The drawing under review shows one solid part. Ordinate dimensions are in mm from its lowest x, y, z. Coordinates: 2 decimals unless noted, no trailing zeros. Write each loop counter-clockwise with the first axis right and the second up, starting at its lowest first coordinate (ties: lowest second). Pieces come first, ordered by that corner, then holes. Notation, with made-up numbers: (4, 59.25) - (38, 59.25) arc R27 cw to (38, 90.25) - close; hole circle Ø11 at (49, 45). An arc over 180 degrees is marked (long way). Use a Markdown table: item, result.
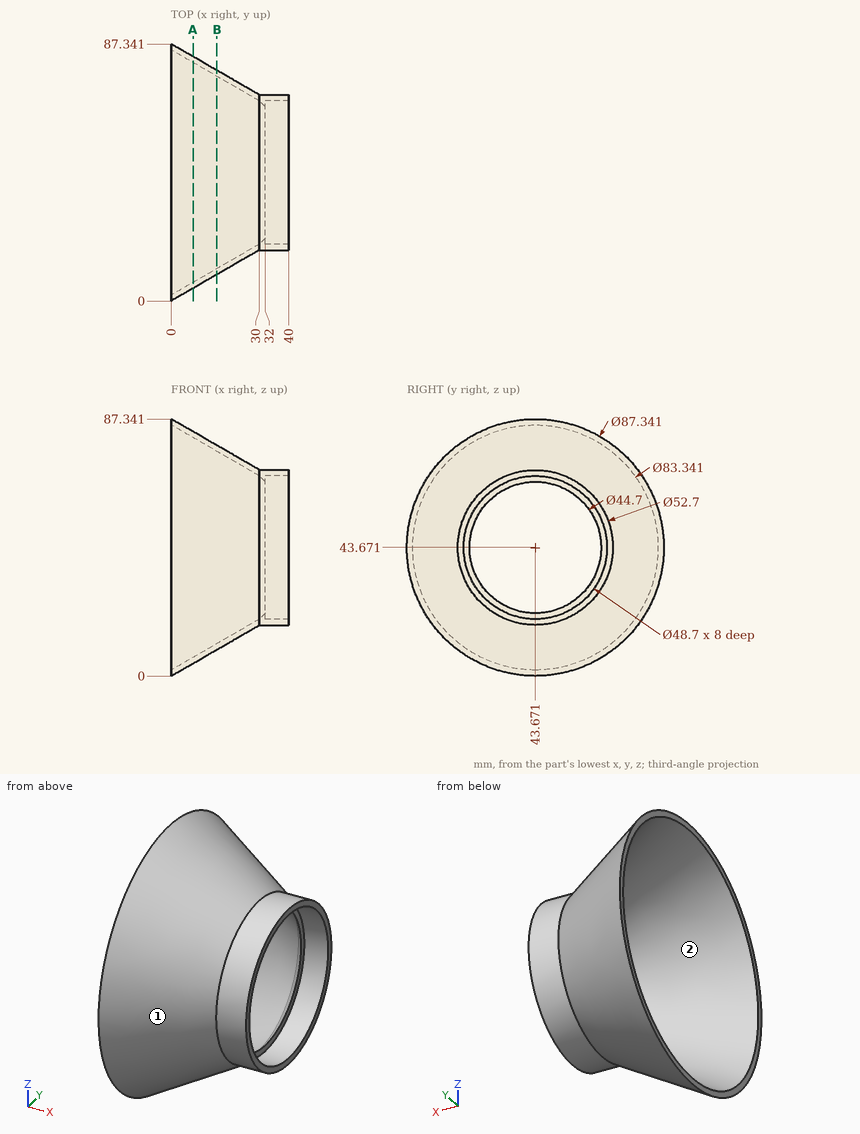
(1) For L1, parallel to Y at x = 12.5, z = 20.5 (1 decimal); L2, parallel to Y at x = 18.5, z = 47; L3, parallel to Z at x = 33, y = 58 (1 decimal), list the stretches that pass through material, from the lowest coordinate up. Write a range as from..to.
Determined:
| item | result |
|---|---|
| L1 | 15.5..18.2, 69.2..71.8 |
| L2 | 10.85..12.86, 74.48..76.49 |
| L3 | 21.6..24, 63.4..65.8 |
(2) Take a section at B-B on x = 15.5. Write out the cut boundary in (y, z).
Determined:
| item | result |
|---|---|
| outline | circle Ø69.44 at (43.67, 43.67); hole circle Ø65.44 at (43.67, 43.67) |
(3) Draft analysis for pull direction Y (two halves, no side actions). For the marked faces 1 and 2, state which applies: +Y half, -Y half, draft (parallel to the pull), parting line (faces both ways), or undercut.
Determined:
| item | result |
|---|---|
| face 1 | parting line |
| face 2 | undercut |
(4) For pin 1 (1.5 mm diameter, centred on x = 10, z = 15.5, fed in from +Y); pin 2 (1 mm diameter, centred on x = 16, y = 22.5, fed in from -Z) (1 decimal); pin 3 (8 mm diameter, centred on x = 27.5, y = 29, fed in from -Z), all flat-tipped, find the tip position at first contact; note any pin that passes through.
Determined:
| item | result |
|---|---|
| pin 1 | y = 70.05 |
| pin 2 | z = 16 |
| pin 3 | z = 16.69 |
(5) Take a section at A-A on x = 7.5. Write out the cut boundary in (y, z).
Determined:
| item | result |
|---|---|
| outline | circle Ø78.68 at (43.67, 43.67); hole circle Ø74.68 at (43.67, 43.67) |
